from build123d import *

# Parameters (mm, degrees)
SKETCH_1_R               = 10
SKETCH_1_R_2             = 1.02
SKETCH_1_R_3             = 1.5
EXTRUDE_1_DEPTH          = 3
SKETCH_2_R               = 5
EXTRUDE_2_DEPTH          = 1
CUT_EXTRUDE_1_DEPTH      = 10
CUT_EXTRUDE_1_DEPTH_BACK = 0.5
SKETCH_3_R               = 3
SKETCH_4_R               = 1.5
CUT_EXTRUDE_2_DEPTH      = 8.5


with BuildPart() as part:
    # ｽｹｯﾁ1 → ﾎﾞｽ - 押し出し1 (new body)
    with BuildSketch(Plane.XY):
        with Locations((-29.978703949, 66)):
            Circle(SKETCH_1_R)
        with Locations((-25.028956481, 61.050252532)):
            Circle(SKETCH_1_R_2, mode=Mode.SUBTRACT)
        with Locations((-29.978703949, 59)):
            Circle(SKETCH_1_R_2, mode=Mode.SUBTRACT)
        with Locations((-34.928451418, 61.050252532)):
            Circle(SKETCH_1_R_2, mode=Mode.SUBTRACT)
        with Locations((-36.978703949, 66)):
            Circle(SKETCH_1_R_2, mode=Mode.SUBTRACT)
        with Locations((-34.928451418, 70.949747468)):
            Circle(SKETCH_1_R_2, mode=Mode.SUBTRACT)
        with Locations((-29.978703949, 73)):
            Circle(SKETCH_1_R_2, mode=Mode.SUBTRACT)
        with Locations((-25.028956481, 70.949747468)):
            Circle(SKETCH_1_R_2, mode=Mode.SUBTRACT)
        with Locations((-22.978703949, 66)):
            Circle(SKETCH_1_R_2, mode=Mode.SUBTRACT)
        with Locations((-29.978703949, 66)):
            Circle(SKETCH_1_R_3, mode=Mode.SUBTRACT)
    extrude(amount=EXTRUDE_1_DEPTH)

    # ｽｹｯﾁ2 → ﾎﾞｽ - 押し出し2 (add)
    with BuildSketch(Plane.XY.offset(3)):
        with Locations((-29.978703949, 66)):
            Circle(SKETCH_2_R)
    extrude(amount=EXTRUDE_2_DEPTH)

    # ｽｹｯﾁ3 → ｶｯﾄ - 押し出し1 (cut, two sides: drawn at the far end of the back side and taken through both)
    with BuildSketch(Plane(origin=(0, 0, 3), x_dir=(-1, 0, 0), z_dir=(0, 0, -1)).offset(-CUT_EXTRUDE_1_DEPTH_BACK)):
        with Locations(Location((29.978703949, 66, 0), (0, 0, 180))):
            Circle(SKETCH_3_R)
    extrude(amount=CUT_EXTRUDE_1_DEPTH + CUT_EXTRUDE_1_DEPTH_BACK, mode=Mode.SUBTRACT)

    # ｽｹｯﾁ4 → ｶｯﾄ - 押し出し2 (cut)
    with BuildSketch(Plane(origin=(0, 0, 3.5), x_dir=(-1, 0, 0), z_dir=(0, 0, -1))):
        with Locations((29.978703949, 66)):
            Circle(SKETCH_4_R)
    extrude(amount=-CUT_EXTRUDE_2_DEPTH, mode=Mode.SUBTRACT)


solid = part.part
Check sheet for the modelled part. Datum: model origin and axes. Units: mm. A direction names the side the tool comes from. Coordinates: 2 decimals unless noted, no trailing zeros. Loops run counter-clockwise (first coordinate to the right, second up) from the corner with the lowest first, then second, coordinate; pieces in that order, holes last. Notation, with made-up numbers: (44.5, 54) -> (64.5, 54) arc R23 cw to (64.5, 82) -> close; hole circle Ø7 at (-13.5, 43.5). An arc over 180 degrees is marked (long way). Answer in a Markdown table with one row per item.
1. Access from +Z, -Z, +X, -X, +Y, -Y to the whole of each face (thin tool, end or side, straight path). Record for faces 4 (the face through (-35, 64, 3)), 5 (the face through (-27.9, 68.4, 0)), 6 (the face through (-27.21, 67.15, 1.77)).
Check values:
| item | result |
|---|---|
| face 4 | +Z |
| face 5 | -Z, +X, -X, +Y, -Y |
| face 6 | -Z |
2. Sectioned sample at D-D, the plane z = 1. Give the number of separate pieces and of enclosed holes in the cut face, then the cut area to 3 significant figures.
Check values:
| item | result |
|---|---|
| separate pieces | 1 |
| enclosed holes | 9 |
| area | 260 mm2 |
3. Go/stop test with flat-tipped pins: pin 1 (1.6 mm diameter, centred on x = -34.93, y = 61.05, fed in from +Z); pin 2 (1 mm diameter, centred on y = 59, z = 1.5, fed in from -X); pin 3 (2 mm diameter, centred on x = -33.5, z = 2.5, fed in from -Y); pin 4 (2 mm diameter, centred on y = 59.5, z = 1, fed in from +X). Record where each tip stops, or that it passes through.
Check values:
| item | result |
|---|---|
| pin 1 | passes through |
| pin 2 | stops at x = -37.58 |
| pin 3 | stops at y = 56.32 |
| pin 4 | stops at x = -21.63 |
4. Material ranges on line 1 along Y through (x, z) = (-24.5, 1.4); line 2 along Y through (x, z) = (-24.25, 0.75); line 3 along X through (y, z) = (71, 1.8), recorded low to high. Write a range as [from, to].
Check values:
| item | result |
|---|---|
| line 1 | y = [57.63, 60.18], [61.92, 70.08], [71.82, 74.37] |
| line 2 | y = [57.8, 60.39], [61.71, 70.29], [71.61, 74.2] |
| line 3 | x = [-38.64, -35.95], [-33.91, -26.05], [-24.01, -21.32] |
5. Sectioned sample at C-C, the plane x = -36.75. Record the boundary of the cut face in (y, z), then the cut area to 3 significant figures.
Check values:
| item | result |
|---|---|
| outline | (58.64, 0) -> (65.01, 0) -> (65.01, 3) -> (58.64, 3) -> close; (66.99, 0) -> (73.36, 0) -> (73.36, 3) -> (66.99, 3) -> close |
| area | 38.2 mm2 |
6. Sectioned sample at A-A, the plane y = 70.5. Record the boundary of the cut face in (x, z), then the cut area to 3 significant figures.
Check values:
| item | result |
|---|---|
| outline | (-38.91, 0) -> (-35.84, 0) -> (-35.84, 3) -> (-38.91, 3) -> close; (-34.01, 0) -> (-25.94, 0) -> (-25.94, 3) -> (-27.8, 3) -> (-27.8, 4) -> (-32.16, 4) -> (-32.16, 3) -> (-34.01, 3) -> close; (-24.11, 0) -> (-21.05, 0) -> (-21.05, 3) -> (-24.11, 3) -> close |
| area | 47.0 mm2 |
7. Release check for a two-part mould opening along X. For faces 1 (the face through (-33.664, 69.379, 3.493)), 2 (the face through (-28.7, 67.3, 3.5)), 3 (the face through (-31.2, 67.2, 4)) record: released by +X, released by -X, zero draft, split by the parting line, or undercut.
Check values:
| item | result |
|---|---|
| face 1 | split by the parting line |
| face 2 | undercut |
| face 3 | zero draft |
8. Sectioned sample at B-B, the plane y = 66. Record the boundary of the cut face in (x, z), then the cut area to 3 significant figures.
Check values:
| item | result |
|---|---|
| outline | (-39.98, 0) -> (-38, 0) -> (-38, 3) -> (-39.98, 3) -> close; (-35.96, 0) -> (-32.98, 0) -> (-32.98, 3.5) -> (-31.48, 3.5) -> (-31.48, 4) -> (-34.98, 4) -> (-34.98, 3) -> (-35.96, 3) -> close; (-28.48, 3.5) -> (-26.98, 3.5) -> (-26.98, 0) -> (-24, 0) -> (-24, 3) -> (-24.98, 3) -> (-24.98, 4) -> (-28.48, 4) -> close; (-21.96, 0) -> (-19.98, 0) -> (-19.98, 3) -> (-21.96, 3) -> close |
| area | 35.3 mm2 |
